Geometry check sheet. Reference: the model listing, model coordinates, mm. Face numbers are marked on the shaded views. A direction names the side the tool comes from. Round coordinates to 2 decimals unless told otherwise and drop trailing zeros. Order: outer loops, then holes, each group sorted by start corner. A loop starts at its lowest first (then second) coordinate and runs counter-clockwise, first axis right, second up. Notation, with made-up numbers: M 10.5,57.5 L 45.5,57.5 A11 cw 45.5,73.5 Z; hole C -5,-21 d1. An arc over 180 degrees is marked long. Answer as a JSON object with one key per item and string values. Group by question number.
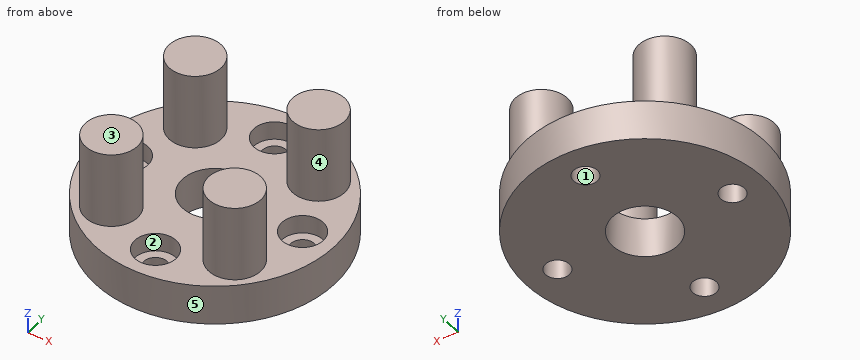
```python
from build123d import *

# Parameters (mm, degrees)
DYNAMIXELHUB_R   = 11
DYNAMIXELHUB_R_2 = 3
DYNAMIXELHUB_R_3 = 1.1
HUB_DEPTH        = 3.7
SKETCH2_R        = 1.9
SCREWSLOT_DEPTH  = 1.7
SCREWSLOTS_COUNT = 4
SKETCH3_R        = 2.4
LEGOPIN_DEPTH    = 7
LEGOPINS_COUNT   = 4


with BuildPart() as part:
    # DynamixelHub → Hub (new body)
    with BuildSketch(Plane.XY):
        Circle(DYNAMIXELHUB_R)
        Circle(DYNAMIXELHUB_R_2, mode=Mode.SUBTRACT)
        with Locations((0, 8)):
            Circle(DYNAMIXELHUB_R_3, mode=Mode.SUBTRACT)
        with Locations((8, 0)):
            Circle(DYNAMIXELHUB_R_3, mode=Mode.SUBTRACT)
        with Locations((0, -8)):
            Circle(DYNAMIXELHUB_R_3, mode=Mode.SUBTRACT)
        with Locations((-8, 0)):
            Circle(DYNAMIXELHUB_R_3, mode=Mode.SUBTRACT)
    extrude(amount=HUB_DEPTH)

    # Sketch2 → ScrewSlot (cut)
    with BuildSketch(Plane.XY.offset(3.7)):
        with Locations((0, 8)):
            Circle(SKETCH2_R)
    screwslot = extrude(amount=-SCREWSLOT_DEPTH, mode=Mode.SUBTRACT)

    # ScrewSlots: ScrewSlot ×4 about axis
    screwslots_axis = Axis((0, 0, 0), (0, 0, 1))
    for i in range(1, SCREWSLOTS_COUNT):
        add(screwslot.rotate(screwslots_axis, i * 360 / SCREWSLOTS_COUNT), mode=Mode.SUBTRACT)

    # Sketch3 → LegoPin (add)
    with BuildSketch(Plane.XY.offset(3.7)):
        with Locations((5.635641046, 5.635641046)):
            Circle(SKETCH3_R)
    legopin = extrude(amount=LEGOPIN_DEPTH)

    # LegoPins: LegoPin ×4 about axis
    legopins_axis = Axis((0, 0, 0), (0, 0, 1))
    for i in range(1, LEGOPINS_COUNT):
        add(legopin.rotate(legopins_axis, i * 360 / LEGOPINS_COUNT))


solid = part.part
```
1) Thickness scan on line 1 along Y through (x, z) = (0, 3); line 2 along Y through (x, z) = (0, 1.9); line 3 along Z through (x, y) = (6.5, 1.25). Record the ranges inside material, lowest first. Write a range as [from, to].
2) Set-up check for the marked faces 1 and 2: record each of +Z, -Z, +X, -X, +Y, -Y from which the full face is reachable in a straight line by a thin tool's end or side.
3) Sectioned sample at D-D (x = -2.25). Record the boundary of the cut face in (y, z), then the cut area to 3 significant figures.
4) Sectioned sample at C-C (z = 2.75). Record the boundary of the cut face in (x, y).
5) Sectioned sample at A-A (y = 0). Record the boundary of the cut face in (x, z), then the cut area to 3 significant figures.
6) Release check for a two-part mould opening along Y. For the marked faces 3, 4 and 5 record: +Y half, -Y half, draft (parallel to the pull), parting line (faces both ways), or undercut.
7) Go/stop test with flat-tipped pins: P1, Ø2, axis at x = 3, z = 8.5, coming from the -Y side; P2, Ø4, axis at x = -7.5, y = 0.5, coming from the +Z side; P3, Ø1, axis at x = 8.5, z = 1, coming from the -Y side; P4, Ø1.3, axis at x = -8, y = 0, coming from the -Z side. Record where each tip stops, or that it passes through.
Final values:
{
 "1": {"line 1": "y = [-11, -9.9], [-6.1, -3], [3, 6.1], [9.9, 11]", "line 2": "y = [-11, -9.1], [-6.9, -3], [3, 6.9], [9.1, 11]", "line 3": "z = [0, 3.7]"},
 "2": {"face 1": "+Z, -Z", "face 2": "+Z"},
 "3": {"outline": "M -10.77,0 L -1.98,0 L -1.98,3.7 L -10.77,3.7 Z; M 1.98,0 L 10.77,0 L 10.77,3.7 L 1.98,3.7 Z", "area": "65.0 mm^2"},
 "4": {"outline": "C 0,0 d22; hole C -8,0 d3.8; hole C 0,0 d6; hole C 0,-8 d3.8; hole C 0,8 d3.8; hole C 8,0 d3.8"},
 "5": {"outline": "M -11,0 L -9.1,0 L -9.1,2 L -9.9,2 L -9.9,3.7 L -11,3.7 Z; M -6.9,0 L -3,0 L -3,3.7 L -6.1,3.7 L -6.1,2 L -6.9,2 Z; M 3,0 L 6.9,0 L 6.9,2 L 6.1,2 L 6.1,3.7 L 3,3.7 Z; M 9.1,0 L 11,0 L 11,3.7 L 9.9,3.7 L 9.9,2 L 9.1,2 Z", "area": "37.5 mm^2"},
 "6": {"face 3": "draft", "face 4": "undercut", "face 5": "parting line"},
 "7": {"P1": "stops at y = -7.39", "P2": "stops at z = 3.7", "P3": "stops at y = -7.55", "P4": "passes through"}
}
